The model under review builds one solid part; all positions refer to its coordinate system, in mm. A direction names the side the tool comes from. Coordinates: 2 decimals unless noted, no trailing zeros. Order: outer loops, then holes, each group sorted by start corner. A loop starts at its lowest first (then second) coordinate and runs counter-clockwise, first axis right, second up. Notation, with made-up numbers: (83.5, -9) -> (88.5, -9) arc R29 ccw to (88.5, 13) -> close; hole circle Ø1 at (43, -20.5). An arc over 180 degrees is marked (long way). Put each result on its own line as item: value.
from build123d import *

# Parameters (mm, degrees)
ESBO_O1_W                = 300
ESBO_O1_H                = 300
ESBO_O1_R                = 5
RESSALTO_EXTRUS_O1_DEPTH = 20
ESBO_O2_W                = 40
ESBO_O2_H                = 40
CORTE_EXTRUS_O1_DEPTH    = 7
ESBO_O3_R                = 5
CORTE_EXTRUS_O2_DEPTH    = 397.948721879


with BuildPart() as part:
    # Esboço1 → Ressalto-extrusão1 (new body)
    with BuildSketch(Plane(origin=(0, 0, 0), x_dir=(1, 0, 0), z_dir=(0, 1, 0))):
        with Locations((124.594594595, -136.351351351)):
            Rectangle(ESBO_O1_W, ESBO_O1_H)
        with Locations(Location((-5.405405405, -6.351351351, 0), (0, 0, 270))):
            Circle(ESBO_O1_R, mode=Mode.SUBTRACT)
        with Locations(Location((254.594594595, -6.351351351, 0), (0, 0, 90))):
            Circle(ESBO_O1_R, mode=Mode.SUBTRACT)
        with Locations(Location((254.594594595, -266.351351351, 0), (0, 0, 270))):
            Circle(ESBO_O1_R, mode=Mode.SUBTRACT)
        with Locations(Location((-5.405405405, -266.351351351, 0), (0, 0, 90))):
            Circle(ESBO_O1_R, mode=Mode.SUBTRACT)
        with Locations(Location((124.594594595, -6.351351351, 0), (0, 0, 90))):
            Circle(ESBO_O1_R, mode=Mode.SUBTRACT)
    extrude(amount=RESSALTO_EXTRUS_O1_DEPTH)

    # Esboço2 → Corte-extrusão1 (cut)
    with BuildSketch(Plane(origin=(0, 20, 0), x_dir=(1, 0, 0), z_dir=(0, 1, 0))):
        with Locations((124.594594595, -136.351351351)):
            Rectangle(ESBO_O2_W, ESBO_O2_H)
    extrude(amount=-CORTE_EXTRUS_O1_DEPTH, mode=Mode.SUBTRACT)

    # Esboço3 → Corte-extrusão2 (cut, through all)
    with BuildSketch(Plane(origin=(0, 13, 0), x_dir=(1, 0, 0), z_dir=(0, 1, 0))):
        with Locations(Location((124.594594595, -136.351351351, 0), (0, 0, 270))):
            Circle(ESBO_O3_R)
    extrude(amount=-CORTE_EXTRUS_O2_DEPTH, mode=Mode.SUBTRACT)


solid = part.part
Item 1: Consider section B-B on z = 150.5. Write out the cut boundary in (x, y), and give its area (3 significant figures).
Answers below:
outline: (-25.41, 0) -> (274.59, 0) -> (274.59, 20) -> (144.59, 20) -> (144.59, 13) -> (104.59, 13) -> (104.59, 20) -> (-25.41, 20) -> close
area: 5,720 mm^2
Item 2: Mouldability with a two-part tool opening along X and no side actions: class faces 1 (the flat face through (144.595, 17, 137)), 2 (the flat face through (274.595, 10, 138)), 3 (the flat face through (122, 0, 101)), 4 (the flat face through (124, 17, 156.351)) as +X half, -X half, draft (parallel to the pull), parting line (faces both ways), or undercut.
Answers below:
face 1: undercut
face 2: +X half
face 3: draft
face 4: undercut
Item 3: For pin 1 Ø6 at (x, z) = (254.59, 266.35) entering from +Y, flat-tipped, find the tip position at first contact; note if it passes through.
Answers below:
pin 1: through
Item 4: For faces 5 (the flat face through (104.595, 17, 137)), 6 (the cylindrical face through (129.476, 9.86, 7.435)), list the 3-axis set-ups (+Z, -Z, +X, -X, +Y, -Y) from which the entire face can be reached by the end or side of a thin tool; tool diameter is ignored.
Answers below:
face 5: +Y
face 6: +Y, -Y
Item 5: For line 1 (X direction, y = 10.5, z = 6); line 2 (X direction, y = 7.25, z = 268); line 3 (Z direction, x = 139.5, y = 15.25), list the stretches that pass through material, from the lowest coordinate up. Write a range as from..to.
Answers below:
line 1: -25.41..-10.39, -0.42..119.61, 129.58..249.61, 259.58..274.59
line 2: -25.41..-10.13, -0.69..249.87, 259.31..274.59
line 3: -13.65..116.35, 156.35..286.35
Item 6: Consider section A-A on x = 133.5. Write out the cut boundary in (y, z), and give its area (3 significant figures).
Answers below:
outline: (0, -13.65) -> (20, -13.65) -> (20, 116.35) -> (13, 116.35) -> (13, 156.35) -> (20, 156.35) -> (20, 286.35) -> (0, 286.35) -> close
area: 5,720 mm^2
Item 7: Consider section C-C on y = 17. Write out the cut boundary in (x, z).
Answers below:
outline: (-25.41, -13.65) -> (274.59, -13.65) -> (274.59, 286.35) -> (-25.41, 286.35) -> close; hole circle Ø10 at (-5.41, 6.35); hole circle Ø10 at (-5.41, 266.35); hole (104.59, 116.35) -> (144.59, 116.35) -> (144.59, 156.35) -> (104.59, 156.35) -> close; hole circle Ø10 at (124.59, 6.35); hole circle Ø10 at (254.59, 6.35); hole circle Ø10 at (254.59, 266.35)
